Autodesk Inventor part; units mm, degrees
ref_plane "YZ Plane" through (0, 0, 0) normal (1, 0, 0) x (0, 1, 0)
ref_plane "XZ Plane" through (0, 0, 0) normal (0, 1, 0) x (-1, 0, 0)
ref_plane "XY Plane" through (0, 0, 0) normal (0, 0, 1) x (1, 0, 0)
sketch "Sketch1" plane through (0, 0, 0) normal (0, 0, 1) x (1, 0, 0)
  line L0 (468.299, -139.1495) -> (-468.299, -139.1495)
  line L1 (-468.299, -139.1495) -> (-468.299, 139.1495)
  line L2 (-468.299, 139.1495) -> (468.299, 139.1495)
  line L3 (468.299, 139.1495) -> (468.299, -139.1495)
  line L4 (468.299, -139.1495) -> (-468.299, 139.1495) construction
  line L5 (-468.299, -139.1495) -> (468.299, 139.1495) construction
  point P0 (0, 0)
  dimension "d0" = 936.598
  dimension "d1" = 278.299
extrude "Plate1" add sketch "Sketch1" along normal blind 1.5
sketch "Sketch2" plane through (-468.299, -137.6495, 1.5) normal (0, -1, 0) x (1, 0, 0)
  line L0 (936.598, 0) -> (0, 0)
  line L1 (0, 0) -> (0, -40)
  line L2 (0, -40) -> (936.598, -40)
  line L3 (936.598, -40) -> (936.598, 0)
edge flange "Flange1" height 40 angle 90 thickness 1.5 bend radius 1.5 thickness toward (0, -1, 0) relief tear relief width 1.5 relief depth 0.75 corner gap 1.5 corner form 2 edges at (0, -139.1495, 0) (-468.299, 0, 0) (0, 139.1495, 0) (468.299, 0, 0) wall of the first edge with corners at (468.299, -137.6495, 1.5) (-468.299, -137.6495, 1.5) (-468.299, -137.6495, -38.5) (468.299, -137.6495, -38.5)
bend "Bend1"
corner "Corner1"
sketch "Sketch3" plane through (-465.7383, -139.1495, -37) normal (0, 0, -1) x (-1, 0, 0)
  line L0 (-931.4767, 0) -> (0, 0)
  line L1 (0, 0) -> (0, 10)
  line L2 (0, 10) -> (-931.4767, 10)
  line L3 (-931.4767, 10) -> (-931.4767, 0)
edge flange "Flange2" height 10 angle 90 thickness 1.5 bend radius 1.5 thickness toward (0, 0, -1) relief tear relief width 1.5 relief depth 0.75 corner gap 1.5 corner form 0 edges at (0, -137.6495, -38.5) (0, 137.6495, -38.5) wall of the first edge with corners at (465.7383, -139.1495, -37) (-465.7383, -139.1495, -37) (-465.7383, -129.1495, -37) (465.7383, -129.1495, -37)
bend "Bend2"
corner "Corner2"
sketch "Sketch4" plane through (0, 0, 1.5) normal (0, 0, 1) x (1, 0, 0)
  circle A0 centre (17.5, -104.6495) radius 2.25
  circle A1 centre (-17.5, -104.6495) radius 2.25
  point P0 (0, 0)
extrude "Extrusion1" cut sketch "Sketch4" against normal through all
equation "\"d3\" = BendReliefWidth"
equation "\"d4\" = BendReliefDepth"
equation "\"d5\" = MinimumRemnant"
equation "\"d6\" = BendRadius"
equation "\"d9\" = BendRadius"
equation "\"d10\" = CornerReliefSize"
equation "\"d11\" = GapSize"
equation "\"d12\" = JacobiRadiusSize"
equation "\"d13\" = BendReliefWidth"
equation "\"d14\" = BendReliefDepth"
equation "\"d15\" = MinimumRemnant"
equation "\"d16\" = BendRadius"
equation "\"d19\" = BendRadius"
equation "\"d20\" = CornerReliefSize"
equation "\"d21\" = GapSize"
equation "\"d22\" = JacobiRadiusSize"
equation "\"BendRadius\" = Thickness"
equation "\"BendReliefWidth\" = Thickness"
equation "\"BendReliefDepth\" = 0.5 * Thickness"
equation "\"CornerReliefSize\" = 4 * Thickness"
equation "\"MinimumRemnant\" = 2 * Thickness"
equation "\"TransitionRadius\" = BendRadius"
equation "\"JacobiRadiusSize\" = BendRadius"
equation "\"GapSize\" = Thickness"
equation "\"d2\" = BendRadius"
properties part number "Base Gabinete" material "Stainless Steel"
For this review, take the finished solid that the model builds, in its own axes (mm). A direction names the side the tool comes from. Give positions to 0.01 mm unless a question says otherwise; leave off trailing zeros. Loops run counter-clockwise (first coordinate to the right, second up) from the corner with the lowest first, then second, coordinate; pieces in that order, holes last.
Item 1: For line 1 along X through (y, z) = (-30.5, -23); line 2 along Y through (x, z) = (-92, -6.5); line 3 along Z through (x, y) = (-133, 127.5), list the stretches that pass through material, from the lowest coordinate up.
Item 2: Tool access review of faces 1 (the flat face through (-7, 2, 1.5)), 2 (the flat face through (7, 137.65, -18)): name each direction out of +Z, -Z, +X, -X, +Y, -Y from which nothing blocks a thin tool from reaching the whole face with its end or side.
Item 3: Take a section at B-B, the plane y = 4. State the section outline as (x, z) points.
Item 4: Take a section at C-C, the plane x = -396. State the section outline as (y, z) points.
Item 5: Draft analysis for pull direction X (two halves, no side actions). For faces 3 (the flat face through (-466.799, 2, -20)), 4 (the flat face through (-7, -137.65, -18)), 5 (the flat face through (466.799, -2, -20)), 6 (the flat face through (-468.299, 2, -20)), state which applies: +X half, -X half, draft (parallel to the pull), parting line (faces both ways), or undercut.
Item 6: Insertion check: pin 1 (12 mm diameter, centred on x = 339, y = -69, fed in from -Z); pin 2 (0.9 mm diameter, centred on x = 466.5, z = 0, fed in from +Y); pin 3 (2.5 mm diameter, centred on x = 467, z = 0, fed in from -Y). Each pin has a flat end and moves straight along its axis. Give the tip position at first contact, or say it passes through.
Item 7: Take a section at A-A, the plane z = -9. State the section outline as (x, y) points.
Calculated:
1. line 1: x = -468.3 to -466.8, 466.8 to 468.3
1. line 2: y = -139.15 to -137.65, 137.65 to 139.15
1. line 3: z = 0 to 1.5
2. face 1: +Z, +X, -X, +Y, -Y
2. face 2: +X, -X
3. outline: (-468.3, -38.5) - (-466.8, -38.5) - (-466.8, -1.5) arc R1.5 cw to (-465.3, 0) - (465.3, 0) arc R1.5 cw to (466.8, -1.5) - (466.8, -38.5) - (468.3, -38.5) - (468.3, -1.5) arc R3 ccw to (465.3, 1.5) - (-465.3, 1.5) arc R3 ccw to (-468.3, -1.5) - close
4. outline: (-139.15, -35.5) arc R3 ccw to (-136.15, -38.5) - (-129.15, -38.5) - (-129.15, -37) - (-136.15, -37) arc R1.5 cw to (-137.65, -35.5) - (-137.65, -1.5) arc R1.5 cw to (-136.15, 0) - (136.15, 0) arc R1.5 cw to (137.65, -1.5) - (137.65, -35.5) arc R1.5 cw to (136.15, -37) - (129.15, -37) - (129.15, -38.5) - (136.15, -38.5) arc R3 ccw to (139.15, -35.5) - (139.15, -1.5) arc R3 ccw to (136.15, 1.5) - (-136.15, 1.5) arc R3 ccw to (-139.15, -1.5) - close
5. face 3: undercut
5. face 4: draft
5. face 5: undercut
5. face 6: -X half
6. pin 1: stops at z = 0
6. pin 2: stops at y = 136.15
6. pin 3: stops at y = -136.15
7. outline: (-468.3, -136.59) - (-466.8, -136.59) - (-466.8, 136.59) - (-468.3, 136.59) - close; (-465.74, -139.15) - (465.74, -139.15) - (465.74, -137.65) - (-465.74, -137.65) - close; (-465.74, 137.65) - (465.74, 137.65) - (465.74, 139.15) - (-465.74, 139.15) - close; (466.8, -136.59) - (468.3, -136.59) - (468.3, 136.59) - (466.8, 136.59) - close
